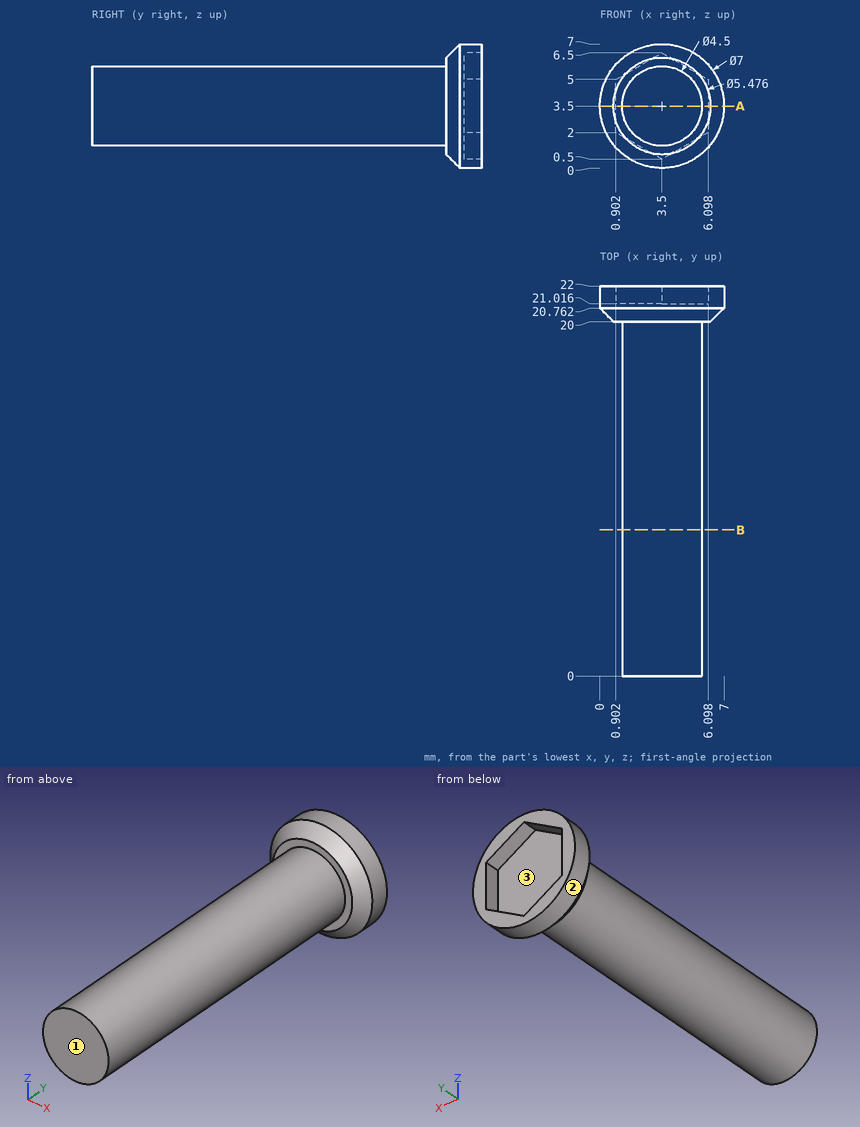
Geometry check sheet. Reference: drawing and pictorial views, mm from the part's lowest x, y, z. Give positions to 0.01 mm unless a question says otherwise; leave off trailing zeros. Order: outer loops, then holes, each group sorted by start corner. A loop starts at its lowest first (then second) coordinate and runs counter-clockwise, first axis right, second up. Notation, with made-up numbers: M -29,-32.5 L -21,-32.5 A18 ccw -21,-1.5 Z; hole C 34,-1.75 d10. An arc over 180 degrees is marked long. Return JSON: item names as keys, results as strings. Group by question number.
1) Section check B-B on y = 8.25. Record the cut outline in (x, z).
2) Section check A-A on z = 3.5. Record the cut outline in (x, y).
3) Go/stop test with flat-tipped pins: pin 1 Ø2 at (x, y) = (6, 8.5) entering from -Z; pin 2 Ø0.5 at (y, z) = (21.5, 3) entering from -X; pin 3 Ø2 at (y, z) = (17.5, 4) entering from -X. Record where each tip stops, or that it passes through.
4) Mould release check, pull along Z, two halves, no side actions. Record for the marked faces 1, 2 and 3: pulls with the +Z half, pulls with the -Z half, needs draft (parallel to the pull), parting line crosses it, or undercut.
5) Scan lines: line 1 (X direction, y = 7, z = 3.5); line 2 (Y direction, x = 3.75, z = 2); line 3 (Z direction, x = 2, y = 17.75). Record each from-to range of solid material in increasing order.
Answer block:
{
 "1": {"outline": "C 3.5,3.5 d4.5"},
 "2": {"outline": "M 0,20.76 L 0.76,20 L 1.25,20 L 1.25,0 L 5.75,0 L 5.75,20 L 6.24,20 L 7,20.76 L 7,22 L 6.1,22 L 6.1,21.02 L 0.9,21.02 L 0.9,22 L 0,22 Z"},
 "3": {"pin 1": "stops at z = 1.82", "pin 2": "stops at x = 0.01", "pin 3": "stops at x = 1.25"},
 "4": {"face 1": "needs draft", "face 2": "parting line crosses it", "face 3": "undercut"},
 "5": {"line 1": "x = 1.25 to 5.75", "line 2": "y = 0 to 21.02", "line 3": "z = 1.82 to 5.18"}
}
